```python
from build123d import *

# Parameters (mm, degrees)
BOSS_EXTRUDE1_DEPTH     = 15
CUT_EXTRUDE1_DEPTH      = 19
CUT_EXTRUDE1_DEPTH_BACK = 26
CUT_EXTRUDE1_START      = -12
SKETCH2_R               = 1.05
FILLET1_R               = 2
SKETCH3_R               = 1.05
BOSS_EXTRUDE2_DEPTH     = 1
CUT_EXTRUDE2_START      = -12
SKETCH2_3_W             = 9.5
SKETCH2_3_H             = 15
SKETCH2_3_R             = 1.05
CUT_EXTRUDE2_DEPTH      = 5
FILLET2_R               = 2
CHAMFER1_SIZE           = 2


with BuildPart() as part:
    # Sketch1 → Boss-Extrude1 (new body)
    with BuildSketch(Plane.XY):
        with BuildLine():
            Line((-16, 12), (-16, 0))
            Line((-16, 0), (-6.5, 0))
            ThreePointArc((-6.5, 0), (0, 6.5), (6.5, 0))
            Line((6.5, 0), (16, 0))
            Line((16, 0), (16, 12))
            Line((16, 12), (-16, 12))
        make_face()
    extrude(amount=BOSS_EXTRUDE1_DEPTH)

    # Sketch2 → Cut-Extrude1 (cut, two sides: drawn at the far end of the back side and taken through both)
    with BuildSketch(Plane.XZ.offset(CUT_EXTRUDE1_START - CUT_EXTRUDE1_DEPTH_BACK)):
        with Locations((-12.25, 7.5)):
            Circle(SKETCH2_R)
        with Locations((12.25, 7.5)):
            Circle(SKETCH2_R)
    extrude(amount=CUT_EXTRUDE1_DEPTH + CUT_EXTRUDE1_DEPTH_BACK, mode=Mode.SUBTRACT)

    # Fillet1
    fillet1_edges = [part.edges().sort_by_distance(p)[0] for p in [
        (16, 6, 15),
        (-16, 6, 15),
        (-16, 6, 0),
        (16, 6, 0),
    ]]
    fillet(fillet1_edges, radius=FILLET1_R)

    # Sketch3 → Boss-Extrude2 (add)
    # profile 1 of 2: a face of its own
    with BuildSketch(Plane.XZ):
        with BuildLine():
            Line((-14, 0), (-6.5, 0))
            Line((-6.5, 0), (-6.5, 15))
            Line((-6.5, 15), (-14, 15))
            ThreePointArc((-14, 15), (-15.414213562, 14.414213562), (-16, 13))
            Line((-16, 13), (-16, 2))
            ThreePointArc((-16, 2), (-15.414213562, 0.585786438), (-14, 0))
        make_face()
        with Locations((-12.25, 7.5)):
            Circle(SKETCH3_R, mode=Mode.SUBTRACT)
    # profile 2 of 2: a face of its own
    with BuildSketch(Plane.XZ):
        with BuildLine():
            Line((6.5, 0), (14, 0))
            ThreePointArc((14, 0), (15.414213562, 0.585786438), (16, 2))
            Line((16, 2), (16, 13))
            ThreePointArc((16, 13), (15.414213562, 14.414213562), (14, 15))
            Line((14, 15), (6.5, 15))
            Line((6.5, 15), (6.5, 0))
        make_face()
        with Locations((12.25, 7.5)):
            Circle(SKETCH3_R, mode=Mode.SUBTRACT)
    extrude(amount=BOSS_EXTRUDE2_DEPTH)

    # Sketch2<3> → Cut-Extrude2 (cut)
    # profile 1 of 2: a face of its own
    with BuildSketch(Plane.XZ.offset(CUT_EXTRUDE2_START)):
        with Locations((-11.25, 7.5)):
            Rectangle(SKETCH2_3_W, SKETCH2_3_H)
        with Locations((-12.25, 7.5)):
            Circle(SKETCH2_3_R, mode=Mode.SUBTRACT)
    # profile 2 of 2: a face of its own
    with BuildSketch(Plane.XZ.offset(CUT_EXTRUDE2_START)):
        with Locations((11.25, 7.5)):
            Rectangle(SKETCH2_3_W, SKETCH2_3_H)
        with Locations((12.25, 7.5)):
            Circle(SKETCH2_3_R, mode=Mode.SUBTRACT)
    extrude(amount=CUT_EXTRUDE2_DEPTH, mode=Mode.SUBTRACT)

    # Fillet2
    fillet2_edges = [part.edges().sort_by_distance(p)[0] for p in [
        (-6.5, 7, 7.5),
        (-6.5, 12, 7.5),
        (6.5, 7, 7.5),
        (6.5, 12, 7.5),
    ]]
    fillet(fillet2_edges, radius=FILLET2_R)

    # Chamfer1
    chamfer1_edges = [part.edges().sort_by_distance(p)[0] for p in [
        (-13.3, 7, 7.5),
        (11.2, 7, 7.5),
    ]]
    chamfer(chamfer1_edges, length=CHAMFER1_SIZE)


solid = part.part
```
Verification items for the finished model (mm, model axes). A direction names the side the tool comes from. Coordinates: 2 decimals unless noted, no trailing zeros. Loops run counter-clockwise (first coordinate to the right, second up) from the corner with the lowest first, then second, coordinate; pieces in that order, holes last. Notation, with made-up numbers: (38, 82) -> (57, 82) arc R26 ccw to (57, 113) -> close; hole circle Ø6 at (33, 80.25). An arc over 180 degrees is marked (long way). Answer in a Markdown table with one row per item. Add a question column.
1. Section check B-B, the plane z = 7.5. Enter the section's corners in (x, y).
2. Draft check along X on faces 4 (the face through (13.25, 2.04, 7.82)), 5 (the face through (-5.93, 11.4, 7.6)), 6 (the face through (0, 12, 7)). Enter one of: +X half, -X half, draft (parallel to the pull), parting line (faces both ways), or undercut.
3. Access from +Z, -Z, +X, -X, +Y, -Y to the whole of each face (thin tool, end or side, straight path). Record for faces 1 (the face through (-6.5, 9.5, 7.4)), 2 (the face through (9, 7, 8)), 3 (the face through (16, 3, 7)).
4. Material ranges on probe 1 along Z at (x, y) = (12.25, 2); probe 2 along X at (y, z) = (9, 11.75); probe 3 along X at (y, z) = (4.5, 4), recorded low to high. Write a range as [from, to].
5. Depth check by flat-ended pin: P1, Ø6, axis at y = 8, z = 5.5, coming from the -X side; P2, Ø2, axis at x = -6, z = 2, coming from the +Y side; P3, Ø0.5, axis at y = 9.5, z = 10, coming from the -X side; P4, Ø6, axis at x = -13.5, z = 5.5, coming from the +Y side. Enter the tip coordinate at first touch or a pass-through.
6. Section check D-D, the plane z = 3.75. Enter the section's corners in (x, y), then the cut area to 3 significant figures.
7. Section check A-A, the plane x = -12.25. Enter the section's corners in (y, z), then the cut area to 3 significant figures.
8. Section check C-C, the plane y = 3. Enter the section's corners in (x, z), then the cut area to 3 significant figures.
Derived:
| question | item | result |
|---|---|---|
| 1 | outline | (-16, -1) -> (-13.3, -1) -> (-13.3, 5) -> (-15.3, 7) -> (-16, 7) -> close; (-11.2, -1) -> (-6.5, -1) -> (-6.5, 0) arc R6.5 cw to (6.5, 0) -> (6.5, -1) -> (11.2, -1) -> (11.2, 5) -> (9.2, 7) -> (8.5, 7) arc R2 cw to (6.5, 9) -> (6.5, 10) arc R2 ccw to (4.5, 12) -> (-4.5, 12) arc R2 ccw to (-6.5, 10) -> (-6.5, 9) arc R2 cw to (-8.5, 7) -> (-9.2, 7) -> (-11.2, 5) -> close; (13.3, -1) -> (16, -1) -> (16, 7) -> (15.3, 7) -> (13.3, 5) -> close |
| 2 | face 4 | undercut |
| 2 | face 5 | -X half |
| 2 | face 6 | draft |
| 3 | face 1 | +Z, -Z, -X, +Y |
| 3 | face 2 | +Z, -Z, +X, +Y |
| 3 | face 3 | +Z, -Z, +X, +Y, -Y |
| 4 | probe 1 | z = [0, 6.45], [8.55, 15] |
| 4 | probe 2 | x = [-6.5, 6.5] |
| 4 | probe 3 | x = [-16, -4.69], [4.69, 16] |
| 5 | P1 | stops at x = -16 |
| 5 | P2 | stops at y = 11.94 |
| 5 | P3 | stops at x = -6.5 |
| 5 | P4 | stops at y = 7 |
| 6 | outline | (-16, -1) -> (-6.5, -1) -> (-6.5, 0) arc R6.5 cw to (6.5, 0) -> (6.5, -1) -> (16, -1) -> (16, 7) -> (8.5, 7) arc R2 cw to (6.5, 9) -> (6.5, 10) arc R2 ccw to (4.5, 12) -> (-4.5, 12) arc R2 ccw to (-6.5, 10) -> (-6.5, 9) arc R2 cw to (-8.5, 7) -> (-16, 7) -> close |
| 6 | area | 242 mm² |
| 7 | outline | (-1, 0) -> (7, 0) -> (7, 4.45) -> (5, 6.45) -> (-1, 6.45) -> close; (-1, 8.55) -> (5, 8.55) -> (7, 10.55) -> (7, 15) -> (-1, 15) -> close |
| 7 | area | 99.2 mm² |
| 8 | outline | (-16, 2) arc R2 ccw to (-14, 0) -> (-5.77, 0) -> (-5.77, 15) -> (-14, 15) arc R2 ccw to (-16, 13) -> close; (5.77, 0) -> (14, 0) arc R2 ccw to (16, 2) -> (16, 13) arc R2 ccw to (14, 15) -> (5.77, 15) -> close; hole circle Ø2.1 at (-12.25, 7.5); hole circle Ø2.1 at (12.25, 7.5) |
| 8 | area | 297 mm² |
